```python
from build123d import *

# Parameters (mm, degrees)
BOSS_EXTRUDE3_DEPTH      = 10
M3_CLEARANCE_HOLE1_D     = 3.6
M3_CLEARANCE_HOLE1_DEPTH = 5.5
M3_CLEARANCE_HOLE1_TIP   = 1.081549114


with BuildPart() as part:
    # Sketch3 → Boss-Extrude3 (new body)
    with BuildSketch(Plane.XY):
        with BuildLine():
            ThreePointArc((10.627637959, -5.374147741), (8.187588203, -0.208463055), (4.251688797, 3.93241088))
            ThreePointArc((4.251688797, 3.93241088), (2.191837366, 4.729023368), (0, 5))
            ThreePointArc((0, 5), (-3.823420235, 3.222026956), (-4.927665225, -0.847416917))
            ThreePointArc((-4.927665225, -0.847416917), (0.77252532, -5.462986054), (7.504596942, -8.374147741))
            ThreePointArc((7.504596942, -8.374147741), (9.507210052, -7.33333117), (10.627637959, -5.374147741))
        make_face()
    extrude(amount=BOSS_EXTRUDE3_DEPTH)

    # M3 Clearance Hole1
    with Locations(Plane(origin=(0, 0, 0), x_dir=(-1, 0, 0), z_dir=(0, 0, -1))):
        with Locations((0, 2)):
            Hole(M3_CLEARANCE_HOLE1_D / 2, depth=M3_CLEARANCE_HOLE1_DEPTH)
            with Locations((0, 0, -(M3_CLEARANCE_HOLE1_DEPTH + M3_CLEARANCE_HOLE1_TIP / 2))):  # 118° drill point
                Cone(0, M3_CLEARANCE_HOLE1_D / 2, M3_CLEARANCE_HOLE1_TIP, mode=Mode.SUBTRACT)


solid = part.part
```
For this review, take the finished solid that the model builds, in its own axes (mm). A direction names the side the tool comes from. Coordinates: 2 decimals unless noted, no trailing zeros. Order: outer loops, then holes, each group sorted by start corner. A loop starts at its lowest first (then second) coordinate and runs counter-clockwise, first axis right, second up. Notation, with made-up numbers: (-32.5, -33) - (0.5, -33) arc R16 ccw to (0.5, -27) - close; hole circle Ø1 at (5.25, 65). An arc over 180 degrees is marked (long way). Answer as a JSON object with one key per item and string values. Group by question number.
1. For probe 1 along X at (y, z) = (2, 1.75); probe 2 along X at (y, z) = (3.25, 1.75); probe 3 along Y at (x, z) = (0.5, 0.75), list the stretches that pass through material, from the lowest coordinate up.
2. Clearance check with flat-ended pins moving along their axes: P1, Ø3, axis at y = -2, z = 7, coming from the -X side; P2, Ø3, axis at y = 2, z = 7, coming from the +X side; P3, Ø1, axis at x = 6, z = 4, coming from the -Y side. State where each tip first meets the part, or that it passes through.
3. The part is to be moulded in two halves that separate along X. For faces 3 (the flat face through (3, -2, 10)), 4 (the conical face through (0.07, 1.69, 6.39)), 5 (the cylindrical face through (-4, 3, 5)), say which applies: pulls with the +X half, pulls with the -X half, needs draft (parallel to the pull), parting line crosses it, or undercut.
4. For faces 1 (the cylindrical face through (-0.234, 3.785, 2.788)), 2 (the cylindrical face through (2.22, 4.72, 4.93)), list the 3-axis set-ups (+Z, -Z, +X, -X, +Y, -Y) from which the entire face can be reached by the end or side of a thin tool; tool diameter is ignored.
5. We need section B-B on y = -0.5. State the section outline as (x, z) points, then the cut area to 3 significant figures.
6. We need section A-A on z = 3. State the section outline as (x, y) points, then the cut area to 3 significant figures.
Final values:
{
 "1": {"probe 1": "-4.58 to -1.8, 1.8 to 6.4", "probe 2": "-3.8 to -1.3, 1.3 to 5.09", "probe 3": "-5.3 to 0.27, 3.73 to 4.99"},
 "2": {"P1": "x = -4.97", "P2": "x = 7.68", "P3": "y = -8.07"},
 "3": {"face 3": "needs draft", "face 4": "undercut", "face 5": "pulls with the -X half"},
 "4": {"face 1": "-Z", "face 2": "+Z, -Z, +X, +Y"},
 "5": {"outline": "(-4.97, 0) - (8.38, 0) - (8.38, 10) - (-4.97, 10) - close", "area": "134 mm²"},
 "6": {"outline": "(-4.93, -0.85) arc R27 ccw to (7.5, -8.37) arc R4 ccw to (10.63, -5.37) arc R18 ccw to (4.25, 3.93) arc R9 ccw to (0, 5) arc R5 ccw to start; hole circle Ø3.6 at (0, 2)", "area": "122 mm²"}
}
